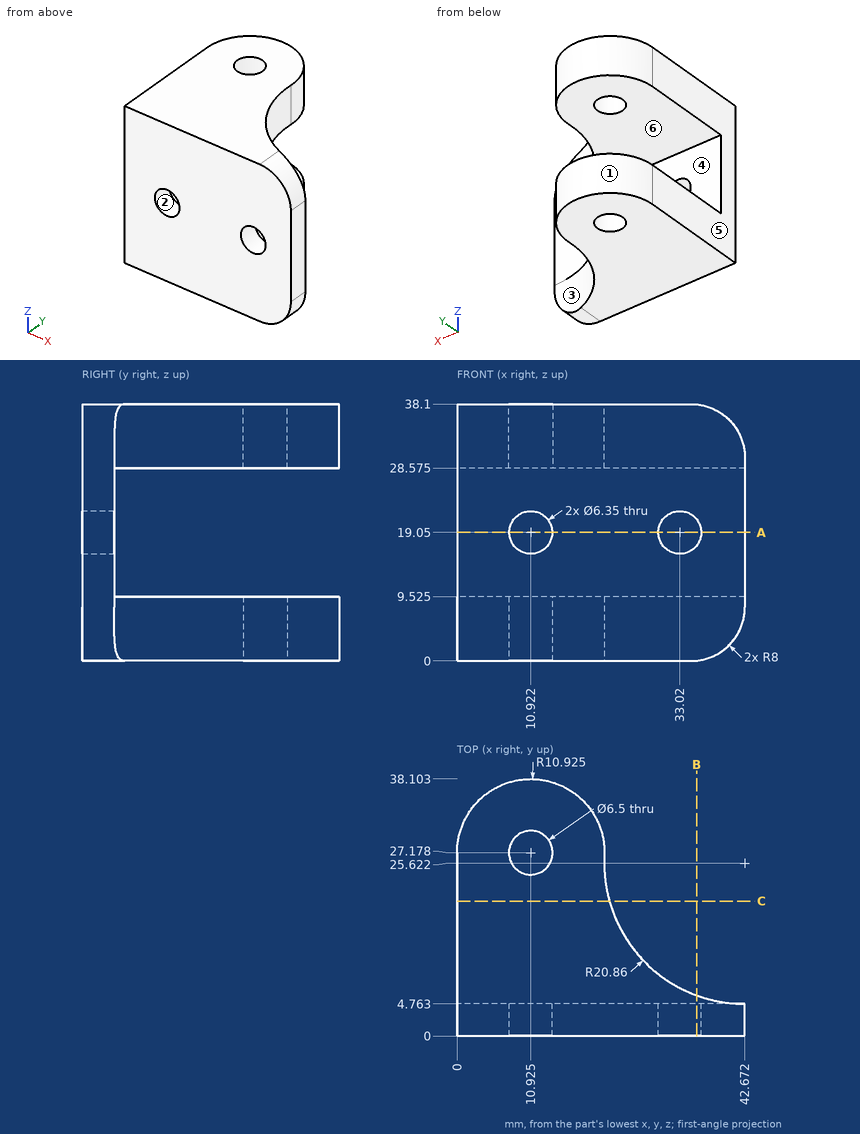
For this review, use the dimensioned drawing (mm, ordinates from the lowest corner) and the shaded views. A direction names the side the tool comes from. Round coordinates to 2 decimals unless told otherwise and drop trailing zeros. Loops run counter-clockwise (first coordinate to the right, second up) from the corner with the lowest first, then second, coordinate; pieces in that order, holes last. Notation, with made-up numbers: M -4.5,-11 L 17.5,-11 A17 cw 17.5,8 Z; hole C 66.25,55 d1. An arc over 180 degrees is marked long. Answer as a JSON object with one key per item and string values.
(1) Take a section at A-A on z = 19.05. Give the boundary of the cut face in (x, y) (1 decimal).
Resolved:
{"outline": "M 0,0 L 7.7,0 L 7.7,4.8 L 0,4.8 Z; M 14.1,0 L 29.8,0 L 29.8,4.8 L 14.1,4.8 Z; M 36.2,0 L 42.7,0 L 42.7,4.8 L 36.2,4.8 Z"}
(2) Take a section at C-C on y = 20. Give the boundary of the cut face in (x, z) (1 decimal).
Resolved:
{"outline": "M 0,0 L 22.6,0 L 22.6,9.5 L 0,9.5 Z; M 0,28.6 L 22.6,28.6 L 22.6,38.1 L 0,38.1 Z"}
(3) Draft analysis for pull direction X (two halves, no side actions). For the marked faces 1, 2, 3 and 4, state which applies: released by +X, released by -X, zero draft, split by the parting line, or undercut.
Resolved:
{"face 1": "split by the parting line", "face 2": "undercut", "face 3": "released by +X", "face 4": "zero draft"}
(4) Clearance check with flat-ended pins moving along their axes: P1, Ø9.5, axis at x = 18.5, z = 23.5, coming from the +Y side; P2, Ø12, axis at x = 25, z = 12, coming from the +Y side (1 decimal); P3, Ø12, axis at y = 30.5, z = 4, coming from the +X side. State where each tip first meets the part, or that it passes through.
Resolved:
{"P1": "y = 4.76", "P2": "y = 33.9", "P3": "x = 21.85"}
(5) Tool access review of the marked faces 5 and 6: name each direction out of +Z, -Z, +X, -X, +Y, -Y from which nothing blocks a thin tool from reaching the whole face with its end or side.
Resolved:
{"face 5": "+Z, -Z, -X, +Y, -Y", "face 6": "+X, -X, +Y"}
(6) To check wall thickness, follow line 1 along X through (y, z) = (1.1, 19.05) (1 decimal); line 2 along Z through (x, y) = (23, 8) (1 decimal); line 3 along Y through (x, z) = (16, 22). State the ranges of each line that lie inside material, in increasing order.
Resolved:
{"line 1": "0 to 7.7, 14.1 to 29.8, 36.2 to 42.7", "line 2": "0 to 9.5, 28.6 to 38.1", "line 3": "0 to 4.76"}
(7) Take a section at B-B on x = 35.5. Give the boundary of the cut face in (y, z) (1 decimal).
Resolved:
{"outline": "M 0,0 L 6,0 L 6,9.5 L 4.8,9.5 L 4.8,17.1 L 0,17.1 Z; M 0,21 L 4.8,21 L 4.8,28.6 L 6,28.6 L 6,38.1 L 0,38.1 Z"}
